For this review, take the finished solid that the model builds, in its own axes (mm). Give positions to 0.01 mm unless a question says otherwise; leave off trailing zeros. Order: outer loops, then holes, each group sorted by start corner. A loop starts at its lowest first (then second) coordinate and runs counter-clockwise, first axis right, second up.
Autodesk Inventor part; units mm, degrees
ref_plane "YZ Plane" through (0, 0, 0) normal (1, 0, 0) x (0, 1, 0)
ref_plane "XZ Plane" through (0, 0, 0) normal (0, 1, 0) x (-1, 0, 0)
ref_plane "XY Plane" through (0, 0, 0) normal (0, 0, 1) x (1, 0, 0)
sketch "Sketch1" plane through (0, 0, 0) normal (0, 1, 0) x (-1, 0, 0)
  point P0 (0, 0)
sketch "Sketch2" plane through (0, 0, 0) normal (0, 1, 0) x (-1, 0, 0)
  circle A0 centre (0, 0) radius 3
  dimension "d0" = 6
extrude "Extrusion1" add sketch "Sketch2" along normal blind 116
sketch "Sketch3" plane through (0, 116, 0) normal (0, 1, 0) x (1, 0, 0)
  circle A0 centre (0, 0) radius 3
extrude "Extrusion2" add sketch "Sketch3" along normal blind 10
sketch "Sketch4" plane through (0, 0, 0) normal (0, -1, 0) x (1, 0, 0)
  circle A0 centre (0, 0) radius 3
  circle A1 centre (0, 0) radius 3
  dimension "d5" = 6
extrude "Extrusion3" add sketch "Sketch4" along normal blind 10
fillet "Fillet1" radius 2 1 edges at (-3, -10, 0)
fillet "Face Fillet1" radius 2 1 edges at (-3, 126, 0)
sketch "Sketch5" plane through (0, 126, 0) normal (0, 1, 0) x (1, 0, 0)
  circle A0 centre (0, 0) radius 3
extrude "Extrusion4" cut sketch "Sketch5" against normal blind 2
sketch "Sketch6" plane through (0, 124, 0) normal (0, 1, 0) x (1, 0, 0)
  circle A0 centre (0, 0) radius 3
extrude "Extrusion5" cut sketch "Sketch6" against normal blind 1
sketch "Sketch7" plane through (0, -10, 0) normal (0, -1, 0) x (1, 0, 0)
  circle A0 centre (0, 0) radius 3
  dimension "d14" = 6
extrude "Extrusion6" cut sketch "Sketch7" against normal blind 3
sketch "Sketch8" plane through (0, -7, 0) normal (0, -1, 0) x (1, 0, 0)
  circle A0 centre (0, 0) radius 3
  dimension "d17" = 6
extrude "Extrusion7" cut sketch "Sketch8" against normal blind 2
sketch "Sketch9" plane through (0, -5, 0) normal (0, -1, 0) x (1, 0, 0)
  circle A0 centre (0, 0) radius 3
  dimension "d20" = 6
extrude "Extrusion8" cut sketch "Sketch9" against normal blind 1
properties material "Gold"
1) To check wall thickness, follow line 1 (Z direction, x = -0.15, y = 50); line 2 (X direction, y = 47, z = 0.25); line 3 (Z direction, x = 1.3, y = 39.5). State the ranges of each line that lie inside material, in increasing order.
Answer sheet:
line 1: z = -3 to 3
line 2: x = -2.99 to 2.99
line 3: z = -2.7 to 2.7
2) Clearance check with flat-ended pins moving along their axes: pin 1 (3 mm diameter, centred on y = 18.5, z = -2, fed in from +X); pin 2 (2 mm diameter, centred on x = 1.5, y = 93, fed in from +Z); pin 3 (1 mm diameter, centred on x = -2, y = 76.5, fed in from -Z). State where each tip first meets the part, or that it passes through.
Answer sheet:
pin 1: stops at x = 2.96
pin 2: stops at z = 2.96
pin 3: stops at z = -2.6
3) We need section A-A on y = 47. Give the boundary of the cut face in (x, z), then the cut area to 3 significant figures.
Answer sheet:
outline: circle Ø6 at (0, 0)
area: 28.3 mm2
